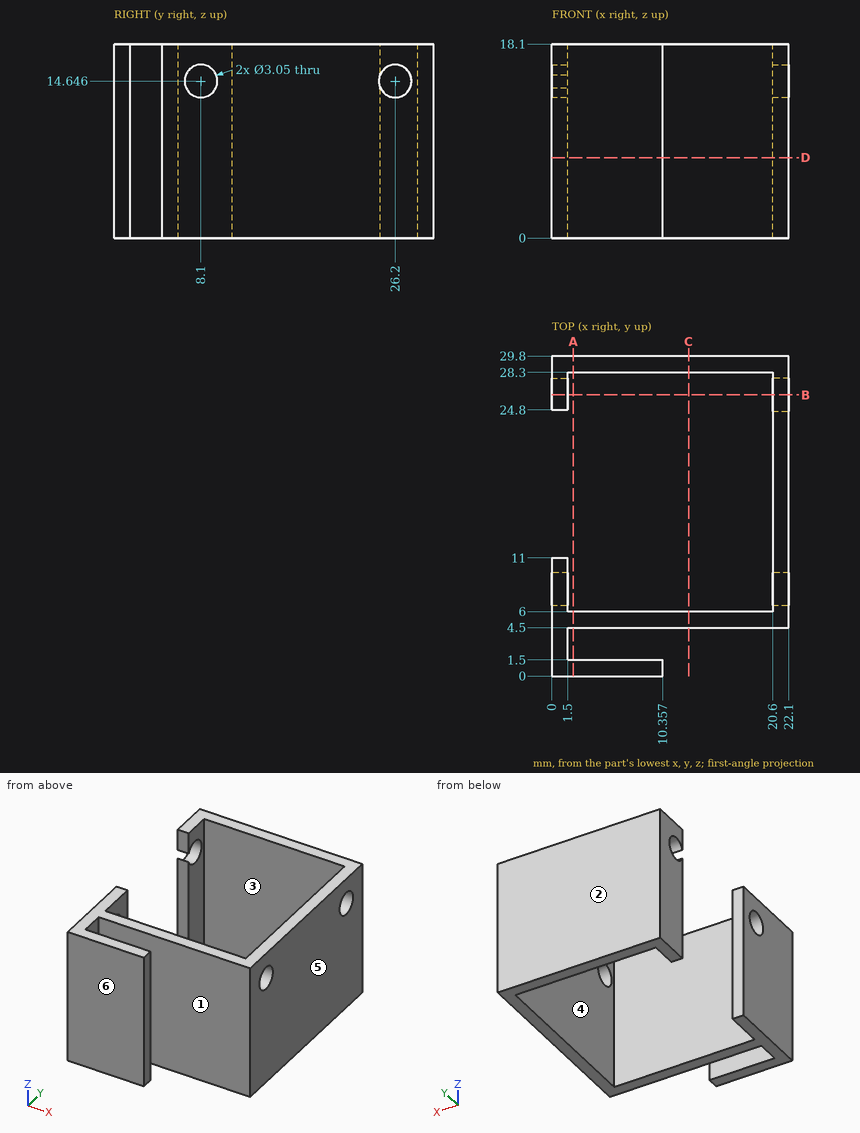
Check sheet for the drawn part. Datum: minimum x, y, z corner. Units: mm. A direction names the side the tool comes from. Round coordinates to 2 decimals unless told otherwise and drop trailing zeros. Order: outer loops, then holes, each group sorted by start corner. A loop starts at its lowest first (then second) coordinate and runs counter-clockwise, first axis right, second up. Notation, with made-up numbers: M -20,3 L 20,3 A5 cw 20,7 Z; hole C 38.25,83 d11. An arc over 180 degrees is marked long. Answer in a Markdown table with one row per item.
(1) Material ranges on line 1 along Y through (x, z) = (10, 7.5); line 2 along Y through (x, z) = (20.5, 17); line 3 along Z through (x, y) = (21.1, 8.1), recorded low to high. Write a range as from..to.
Findings:
| item | result |
|---|---|
| line 1 | y = 0..1.5, 4.5..6, 28.3..29.8 |
| line 2 | y = 4.5..6, 28.3..29.8 |
| line 3 | z = 0..13.12, 16.17..18.1 |
(2) Section check D-D on z = 7.5. Record the boundary of the cut face in (x, y).
Findings:
| item | result |
|---|---|
| outline | M 0,0 L 10.36,0 L 10.36,1.5 L 1.5,1.5 L 1.5,4.5 L 22.1,4.5 L 22.1,29.8 L 0,29.8 L 0,24.8 L 1.5,24.8 L 1.5,28.3 L 20.6,28.3 L 20.6,6 L 1.5,6 L 1.5,11 L 0,11 Z |
(3) Gauge pin test, flat ends, axial feed: pin 1 (1.2 mm diameter, centred on y = 0.5, z = 11, fed in from +X); pin 2 (3 mm diameter, centred on y = 15, z = 4.5, fed in from -X); pin 3 (1.5 mm diameter, centred on y = 3.5, z = 10, fed in from +X). Record the tip position at first contact, or that the pin passes through.
Findings:
| item | result |
|---|---|
| pin 1 | stops at x = 10.36 |
| pin 2 | stops at x = 20.6 |
| pin 3 | stops at x = 1.5 |
(4) Draft check along Y on the marked faces 4, 5 and 6. Enter one of: +Y half, -Y half, draft (parallel to the pull), parting line (faces both ways), or undercut.
Findings:
| item | result |
|---|---|
| face 4 | undercut |
| face 5 | draft |
| face 6 | -Y half |
(5) Set-up check for the marked faces 1, 2 and 3: record each of +Z, -Z, +X, -X, +Y, -Y from which the full face is reachable in a straight line by a thin tool's end or side.
Findings:
| item | result |
|---|---|
| face 1 | +Z, -Z, +X |
| face 2 | +Z, -Z, +X, -X, +Y |
| face 3 | +Z, -Z |
(6) Section check A-A on x = 2. Record the boundary of the cut face in (y, z).
Findings:
| item | result |
|---|---|
| outline | M 0,0 L 1.5,0 L 1.5,18.1 L 0,18.1 Z; M 4.5,0 L 6,0 L 6,18.1 L 4.5,18.1 Z; M 28.3,0 L 29.8,0 L 29.8,18.1 L 28.3,18.1 Z |
(7) Section check B-B on y = 26.2. Record the boundary of the cut face in (x, z).
Findings:
| item | result |
|---|---|
| outline | M 0,0 L 1.5,0 L 1.5,13.12 L 0,13.12 Z; M 0,16.17 L 1.5,16.17 L 1.5,18.1 L 0,18.1 Z; M 20.6,0 L 22.1,0 L 22.1,13.12 L 20.6,13.12 Z; M 20.6,16.17 L 22.1,16.17 L 22.1,18.1 L 20.6,18.1 Z |
(8) Section check C-C on x = 12.75. Record the boundary of the cut face in (y, z), plus the area to 3 significant figures.
Findings:
| item | result |
|---|---|
| outline | M 4.5,0 L 6,0 L 6,18.1 L 4.5,18.1 Z; M 28.3,0 L 29.8,0 L 29.8,18.1 L 28.3,18.1 Z |
| area | 54.3 mm^2 |
